from build123d import *

# Parameters (mm, degrees)
F1_DEPTH      = 500
F3_DEPTH      = 500.001
F5_DEPTH      = 25.001
F5_DEPTH_BACK = 25
F7_D          = 9


with BuildPart() as f1:
    # F0 (on Top) → F1 (new body)
    with BuildSketch(Plane.XY):
        with BuildLine():
            ThreePointArc((25, 20), (23.5355339059, 23.5355339059), (20, 25))
            Line((20, 25), (-20, 25))
            ThreePointArc((-20, 25), (-23.5355339059, 23.5355339059), (-25, 20))
            Line((-25, 20), (-25, -20))
            ThreePointArc((-25, -20), (-23.5355339059, -23.5355339059), (-20, -25))
            Line((-20, -25), (20, -25))
            ThreePointArc((20, -25), (23.5355339059, -23.5355339059), (25, -20))
            Line((25, -20), (25, 20))
        make_face()
    extrude(amount=F1_DEPTH)

    # F2 (on face) → F3 (cut, through all)
    with BuildSketch(Plane.XY.offset(500)):
        with BuildLine():
            ThreePointArc((-22, -20), (-21.4142135624, -21.4142135624), (-20, -22))
            Line((-20, -22), (20, -22))
            ThreePointArc((20, -22), (21.4142135624, -21.4142135624), (22, -20))
            Line((22, -20), (22, 20))
            ThreePointArc((22, 20), (21.4142135624, 21.4142135624), (20, 22))
            Line((20, 22), (-20, 22))
            ThreePointArc((-20, 22), (-21.4142135624, 21.4142135624), (-22, 20))
            Line((-22, 20), (-22, -20))
        make_face()
    extrude(amount=-F3_DEPTH, mode=Mode.SUBTRACT)

    # F4 (on Right) → F5 (cut, two sides)
    with BuildSketch(Plane.YZ) as f5_sk:
        Polygon((25, 500), (-25, 500), (25, 450), align=None)
    extrude(amount=-F5_DEPTH, mode=Mode.SUBTRACT)
    extrude(f5_sk.sketch, amount=F5_DEPTH_BACK, mode=Mode.SUBTRACT)

    # F7 (through all)
    with Locations(Plane.YZ.offset(25)):
        with Locations((0, 50)):
            Hole(F7_D / 2)


solid = f1.part
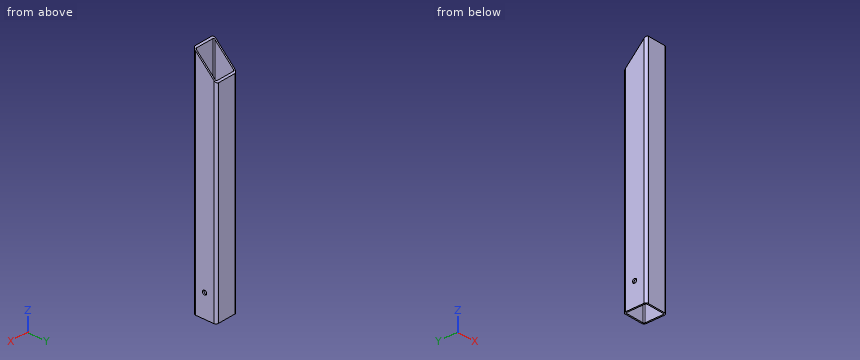
Source: CAD feature listing. Evaluate the final solid. Frame: model axes, mm. Give positions to 0.01 mm unless a question says otherwise; leave off trailing zeros. Order: outer loops, then holes, each group sorted by start corner. A loop starts at its lowest first (then second) coordinate and runs counter-clockwise, first axis right, second up. Notation, with made-up numbers: (-36, 74) -> (-10, 74) arc R20 cw to (-10, 86) -> close; hole circle Ø2 at (27.25, 11). An arc over 180 degrees is marked (long way). Write item = value, one per line.
Item 1: Section query D-D (z = 180.5). Output: boundary loops of the cut face in (x, y), then the cut area to 3 significant figures.
Check result:
outline = (-25, -20) arc R5 ccw to (-20, -25) -> (20, -25) arc R5 ccw to (25, -20) -> (25, 20) arc R5 ccw to (20, 25) -> (-20, 25) arc R5 ccw to (-25, 20) -> close; hole (-22, -20) arc R2 ccw to (-20, -22) -> (20, -22) arc R2 ccw to (22, -20) -> (22, 20) arc R2 ccw to (20, 22) -> (-20, 22) arc R2 ccw to (-22, 20) -> close
area = 546 mm²
Item 2: Section query C-C (x = 14). Output: boundary loops of the cut face in (y, z), then the cut area to 3 significant figures.
Check result:
outline = (-25, 0) -> (-22, 0) -> (-22, 497) -> (-25, 500) -> close; (22, 0) -> (25, 0) -> (25, 450) -> (22, 453) -> close
area = 2,850 mm²
Item 3: Section query A-A (y = 0). Output: boundary loops of the cut face in (x, z), then the cut area to 3 significant figures.
Check result:
outline = (-25, 0) -> (-22, 0) -> (-22, 45.5) -> (-25, 45.5) -> close; (-25, 54.5) -> (-22, 54.5) -> (-22, 475) -> (-25, 475) -> close; (22, 0) -> (25, 0) -> (25, 45.5) -> (22, 45.5) -> close; (22, 54.5) -> (25, 54.5) -> (25, 475) -> (22, 475) -> close
area = 2,800 mm²
Item 4: Section query B-B (z = 50). Output: boundary loops of the cut face in (x, y).
Check result:
outline = (-25, -20) arc R5 ccw to (-20, -25) -> (20, -25) arc R5 ccw to (25, -20) -> (25, -4.5) -> (22, -4.5) -> (22, -20) arc R2 cw to (20, -22) -> (-20, -22) arc R2 cw to (-22, -20) -> (-22, -4.5) -> (-25, -4.5) -> close; (-25, 4.5) -> (-22, 4.5) -> (-22, 20) arc R2 cw to (-20, 22) -> (20, 22) arc R2 cw to (22, 20) -> (22, 4.5) -> (25, 4.5) -> (25, 20) arc R5 ccw to (20, 25) -> (-20, 25) arc R5 ccw to (-25, 20) -> close
Item 5: Ray query, probe 1 along Y at (x, z) = (6, 418); probe 2 along Z at (x, y) = (-23.9, 0). Return the intervals inside material, ascending.
Check result:
probe_1 = -25 to -22, 22 to 25
probe_2 = 0 to 45.5, 54.5 to 475
